The model under review builds one solid part; all positions refer to its coordinate system, in mm. Coordinates: 2 decimals unless noted, no trailing zeros. Write each loop counter-clockwise with the first axis right and the second up, starting at its lowest first coordinate (ties: lowest second). Pieces come first, ordered by that corner, then holes. Notation, with made-up numbers: (68.25, -12) -> (104.25, -12) arc R22 cw to (104.25, 12) -> close; hole circle Ø1 at (54.25, 2). An arc over 180 degrees is marked (long way). Put each result on its own line as item: value. Start each with the question number.
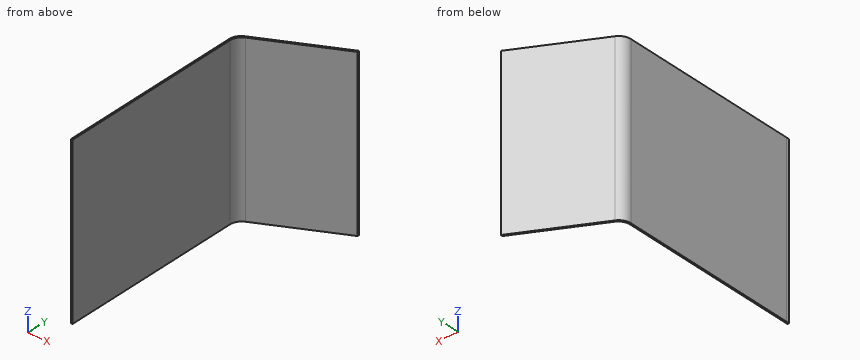
from build123d import *

# Parameters (mm, degrees)
BOSS_EXTRUDE1_DEPTH = 280


with BuildPart() as part:
    # Sketch1 → Boss-Extrude1 (new body)
    with BuildSketch(Plane.XY):
        with BuildLine():
            Line((-6.985, -1.5), (-6.985, 0))
            Line((-6.985, 0), (-6.985, 1.5))
            Line((-6.985, 1.5), (-141.773150354, -69.150147775))
            ThreePointArc((-141.773150354, -69.150147775), (-149.738239599, -76.743206199), (-152.480995182, -87.400338774))
            Line((-152.480995182, -87.400338774), (-144.05, -401.823477062))
            Line((-144.05, -401.823477062), (-144.05, -407.15))
            Line((-144.05, -407.15), (-141.05, -407.15))
            Line((-141.05, -407.15), (-149.573857666, -89.263674623))
            ThreePointArc((-149.573857666, -89.263674623), (-146.831102083, -78.606542048), (-138.866012838, -71.013483624))
            Line((-138.866012838, -71.013483624), (-6.985, -1.887132226))
            Line((-6.985, -1.887132226), (-6.985, -1.5))
        make_face()
    extrude(amount=-BOSS_EXTRUDE1_DEPTH)


solid = part.part
1. Wall thickness on line 1 (X direction, y = -285.5, z = -109.5); line 2 (X direction, y = -65, z = -102); line 3 (Y direction, x = -14, z = -77): over which ranges is each line inside the solid? List them lowest first. Write a range as from..to.
2. Consider section C-C on x = -20.5. State the section outline as (y, z) points, then the cut area to 3 significant figures.
3. Consider section B-B on y = -155. State the section outline as (x, z) points.
4. Insertion check: P1, Ø1, axis at x = -52, z = -234, coming from the -Y side; P2, Ø5, axis at y = -298.5, z = -210, coming from the +X side; P3, Ø3, axis at y = -190.5, z = -82.5, coming from the -X side. Each pin has a flat end and moves straight along its axis. Give the tip position at first contact, or say it passes through.
5. Consider section A-A on z = -80. State the section outline as (x, y) points (3 decimals).
Output values:
1. line 1: x = -147.17..-144.31
1. line 2: x = -133.86..-127.39
1. line 3: y = -5.56..-2.18
2. outline: (-8.97, -280) -> (-5.58, -280) -> (-5.58, 0) -> (-8.97, 0) -> close
2. area: 948 mm^2
3. outline: (-150.67, -280) -> (-147.81, -280) -> (-147.81, 0) -> (-150.67, 0) -> close
4. P1: stops at y = -25.74
4. P2: stops at x = -143.9
4. P3: stops at x = -149.76
5. outline: (-152.481, -87.4) -> (-144.05, -401.823) -> (-144.05, -407.15) -> (-141.05, -407.15) -> (-149.574, -89.264) arc R20 cw to (-138.866, -71.013) -> (-6.985, -1.887) -> (-6.985, 1.5) -> (-141.773, -69.15) arc R20 ccw to start
